from build123d import *

# Parameters (mm, degrees)
SKETCH1_R                  = 5.25
SKETCH1_R_2                = 2.5
BOSS_EXTRUDE1_DEPTH        = 1.6
SKETCH3_W                  = 120
SKETCH3_H                  = 1.6
BOSS_EXTRUDE3_DEPTH        = 60
SKETCH4_R                  = 3
SKETCH4_R_2                = 1.55
SKETCH4_R_3                = 1.75
CUT_EXTRUDE1_DEPTH         = 10
SKETCH6_R                  = 1.7
CUT_EXTRUDE2_DEPTH         = 25
CONVERT_SOLID1_START       = -61
CONVERT_SOLID1_DEPTH       = 122
CONVERT_SOLID1_START_2     = -60
CONVERT_SOLID1_2_DEPTH     = 120
CUT_EXTRUDE3_OUTLINE_W     = 120
CUT_EXTRUDE3_OUTLINE_H     = 60
CUT_EXTRUDE3_OUTLINE_R     = 1.7
CUT_EXTRUDE3_OUTLINE_R_2   = 1.55
CUT_EXTRUDE3_OUTLINE_R_3   = 1.75
CUT_EXTRUDE3_OUTLINE_R_4   = 3
CUT_EXTRUDE3_DEPTH         = 32
CUT_EXTRUDE3_START         = -1.6
CUT_EXTRUDE3_2_OUTLINE_W   = 23.75
CUT_EXTRUDE3_2_OUTLINE_H   = 1.229203673
CUT_EXTRUDE3_2_DEPTH       = 1.6
CUT_EXTRUDE3_3_OUTLINE_W   = 120
CUT_EXTRUDE3_3_OUTLINE_H   = 122.283185308
CUT_EXTRUDE3_3_OUTLINE_W_2 = 23.75
CUT_EXTRUDE3_3_OUTLINE_H_2 = 26.1
CUT_EXTRUDE3_3_OUTLINE_R   = 2.5
CUT_EXTRUDE3_3_OUTLINE_R_2 = 5.25
CUT_EXTRUDE3_3_OUTLINE_R_3 = 1.7
CUT_EXTRUDE3_3_OUTLINE_R_4 = 1.55
CUT_EXTRUDE3_3_OUTLINE_R_5 = 1.75
CUT_EXTRUDE3_3_OUTLINE_R_6 = 3
CUT_EXTRUDE3_3_DEPTH       = 1.6


with BuildPart() as part:
    # Sketch1 → Boss-Extrude1 (new body)
    with BuildSketch(Plane(origin=(0, 0, 0), x_dir=(1, 0, 0), z_dir=(0, 1, 0))):
        Polygon((-60, -12), (-60, 20), (60, 20), (60, -12), (34.5, -12), (11, -12), align=None)
        with Locations(Location((0, 0, 0), (0, 0, 270))):
            Circle(SKETCH1_R, mode=Mode.SUBTRACT)
        with Locations(Location((-43, 0, 0), (0, 0, 270))):
            Circle(SKETCH1_R_2, mode=Mode.SUBTRACT)
        with Locations(Location((43, 0, 0), (0, 0, 90))):
            Circle(SKETCH1_R_2, mode=Mode.SUBTRACT)
    boss_extrude1 = extrude(amount=BOSS_EXTRUDE1_DEPTH)

    # Sketch3 → Boss-Extrude3 (add)
    with BuildSketch(Plane.XZ):
        with Locations((0, 12.8)):
            Rectangle(SKETCH3_W, SKETCH3_H)
    extrude(amount=-BOSS_EXTRUDE3_DEPTH)

    # Mirror1: Boss-Extrude1 across plane
    add(boss_extrude1.mirror(Plane.ZX.offset(30)))

    # Sketch4 → Cut-Extrude1 (cut)
    with BuildSketch(Plane.XY.offset(12)):
        with Locations(Location((22.75, 26.5, 0), (0, 0, 180))):
            Circle(SKETCH4_R)
        with Locations(Location((31.5, 6.5, 0), (0, 0, 180))):
            Circle(SKETCH4_R_2)
        with Locations(Location((14, 6.5, 0), (0, 0, 180))):
            Circle(SKETCH4_R_2)
        with Locations(Location((22.75, 15, 0), (0, 0, 180))):
            Circle(SKETCH4_R_3)
    extrude(amount=CUT_EXTRUDE1_DEPTH, mode=Mode.SUBTRACT)

    # Sketch6 → Cut-Extrude2 (cut)
    with BuildSketch(Plane(origin=(124.244525073, 40.7, 12), x_dir=(1, 0, 0), z_dir=(0, 0, 1))):
        with Locations(Location((-175.244525073, 9.7, 0), (0, 0, 180))):
            Circle(SKETCH6_R)
        with Locations(Location((-146.994525073, 9.7, 0), (0, 0, 180))):
            Circle(SKETCH6_R)
        with Locations(Location((-101.494525073, 9.7, 0), (0, 0, 180))):
            Circle(SKETCH6_R)
        with Locations(Location((-73.244525073, 9.7, 0), (0, 0, 180))):
            Circle(SKETCH6_R)
        with Locations((-175.244525073, -34.5)):
            Circle(SKETCH6_R)
        with Locations((-146.994525073, -34.5)):
            Circle(SKETCH6_R)
        with Locations(Location((-101.494525073, -34.5, 0), (0, 0, 180))):
            Circle(SKETCH6_R)
        with Locations(Location((-73.244525073, -34.5, 0), (0, 0, 180))):
            Circle(SKETCH6_R)
    extrude(amount=CUT_EXTRUDE2_DEPTH, mode=Mode.SUBTRACT)

    # Convert-Solid1: read off the stored shape, not the designer's step
    # Convert-Solid1 outline → Convert-Solid1 (cut)
    with BuildSketch(Plane.YZ.offset(CONVERT_SOLID1_START)):
        with BuildLine():
            Line((60, 13.6), (57.2, 13.6))
            ThreePointArc((57.2, 13.6), (59.179898987, 12.779898987), (60, 10.8))
            Line((60, 10.8), (60, 13.6))
        make_face()
        with BuildLine():
            ThreePointArc((0, 10.8), (0.820101013, 12.779898987), (2.8, 13.6))
            Line((2.8, 13.6), (0, 13.6))
            Line((0, 13.6), (0, 10.8))
        make_face()
    extrude(amount=CONVERT_SOLID1_DEPTH, mode=Mode.SUBTRACT)

    # Convert-Solid1 2 outline → Convert-Solid1 2 (add)
    with BuildSketch(Plane.YZ.offset(CONVERT_SOLID1_START_2)):
        with BuildLine():
            Line((58.4, 12), (57.2, 12))
            ThreePointArc((57.2, 12), (58.048528137, 11.648528137), (58.4, 10.8))
            Line((58.4, 10.8), (58.4, 12))
        make_face()
        with BuildLine():
            ThreePointArc((1.6, 10.8), (1.951471863, 11.648528137), (2.8, 12))
            Line((2.8, 12), (1.6, 12))
            Line((1.6, 12), (1.6, 10.8))
        make_face()
    extrude(amount=CONVERT_SOLID1_2_DEPTH)

    # Cut-Extrude3: read off the stored shape, not the designer's step
    # Cut-Extrude3 outline → Cut-Extrude3 (cut)
    with BuildSketch(Plane(origin=(0, 0, 12), x_dir=(-1, 0, 0), z_dir=(0, 0, -1))):
        with Locations((0, 30)):
            Rectangle(CUT_EXTRUDE3_OUTLINE_W, CUT_EXTRUDE3_OUTLINE_H)
        with Locations((51, 50.4)):
            Circle(CUT_EXTRUDE3_OUTLINE_R, mode=Mode.SUBTRACT)
        with Locations((-51, 6.2)):
            Circle(CUT_EXTRUDE3_OUTLINE_R, mode=Mode.SUBTRACT)
        with Locations((-31.5, 6.5)):
            Circle(CUT_EXTRUDE3_OUTLINE_R_2, mode=Mode.SUBTRACT)
        with Locations((-22.75, 6.2)):
            Circle(CUT_EXTRUDE3_OUTLINE_R, mode=Mode.SUBTRACT)
        with Locations((-14, 6.5)):
            Circle(CUT_EXTRUDE3_OUTLINE_R_2, mode=Mode.SUBTRACT)
        with Locations((-22.75, 15)):
            Circle(CUT_EXTRUDE3_OUTLINE_R_3, mode=Mode.SUBTRACT)
        with Locations((-22.75, 26.5)):
            Circle(CUT_EXTRUDE3_OUTLINE_R_4, mode=Mode.SUBTRACT)
        with Locations((22.75, 6.2)):
            Circle(CUT_EXTRUDE3_OUTLINE_R, mode=Mode.SUBTRACT)
        with Locations((51, 6.2)):
            Circle(CUT_EXTRUDE3_OUTLINE_R, mode=Mode.SUBTRACT)
        with Locations((-51, 50.4)):
            Circle(CUT_EXTRUDE3_OUTLINE_R, mode=Mode.SUBTRACT)
        with Locations((-22.75, 50.4)):
            Circle(CUT_EXTRUDE3_OUTLINE_R, mode=Mode.SUBTRACT)
        with Locations((22.75, 50.4)):
            Circle(CUT_EXTRUDE3_OUTLINE_R, mode=Mode.SUBTRACT)
    extrude(amount=CUT_EXTRUDE3_DEPTH, mode=Mode.SUBTRACT)

    # Cut-Extrude3 2 outline → Cut-Extrude3 2 (cut)
    with BuildSketch(Plane(origin=(0, 0, 12), x_dir=(-1, 0, 0), z_dir=(0, 0, -1)).offset(CUT_EXTRUDE3_START)):
        with Locations((-22.625, 0.614601836)):
            Rectangle(CUT_EXTRUDE3_2_OUTLINE_W, CUT_EXTRUDE3_2_OUTLINE_H)
    extrude(amount=CUT_EXTRUDE3_2_DEPTH, mode=Mode.SUBTRACT)

    # Cut-Extrude3 3 outline → Cut-Extrude3 3 (add)
    with BuildSketch(Plane(origin=(0, 0, 12), x_dir=(-1, 0, 0), z_dir=(0, 0, -1)).offset(CUT_EXTRUDE3_START)):
        with Locations((0, 30)):
            Rectangle(CUT_EXTRUDE3_3_OUTLINE_W, CUT_EXTRUDE3_3_OUTLINE_H)
        with Locations((-22.625, -11.820796327)):
            Rectangle(CUT_EXTRUDE3_3_OUTLINE_W_2, CUT_EXTRUDE3_3_OUTLINE_H_2, mode=Mode.SUBTRACT)
        with Locations((-43, -11.141592654)):
            Circle(CUT_EXTRUDE3_3_OUTLINE_R, mode=Mode.SUBTRACT)
        with Locations((0, -11.141592654)):
            Circle(CUT_EXTRUDE3_3_OUTLINE_R_2, mode=Mode.SUBTRACT)
        with Locations((43, -11.141592654)):
            Circle(CUT_EXTRUDE3_3_OUTLINE_R, mode=Mode.SUBTRACT)
        with Locations((51, 50.4)):
            Circle(CUT_EXTRUDE3_3_OUTLINE_R_3, mode=Mode.SUBTRACT)
        with Locations((-51, 6.2)):
            Circle(CUT_EXTRUDE3_3_OUTLINE_R_3, mode=Mode.SUBTRACT)
        with Locations((-31.5, 6.5)):
            Circle(CUT_EXTRUDE3_3_OUTLINE_R_4, mode=Mode.SUBTRACT)
        with Locations((-22.75, 6.2)):
            Circle(CUT_EXTRUDE3_3_OUTLINE_R_3, mode=Mode.SUBTRACT)
        with Locations((-14, 6.5)):
            Circle(CUT_EXTRUDE3_3_OUTLINE_R_4, mode=Mode.SUBTRACT)
        with Locations((-22.75, 15)):
            Circle(CUT_EXTRUDE3_3_OUTLINE_R_5, mode=Mode.SUBTRACT)
        with Locations((-22.75, 26.5)):
            Circle(CUT_EXTRUDE3_3_OUTLINE_R_6, mode=Mode.SUBTRACT)
        with Locations((22.75, 6.2)):
            Circle(CUT_EXTRUDE3_3_OUTLINE_R_3, mode=Mode.SUBTRACT)
        with Locations((51, 6.2)):
            Circle(CUT_EXTRUDE3_3_OUTLINE_R_3, mode=Mode.SUBTRACT)
        with Locations((-51, 50.4)):
            Circle(CUT_EXTRUDE3_3_OUTLINE_R_3, mode=Mode.SUBTRACT)
        with Locations((-22.75, 50.4)):
            Circle(CUT_EXTRUDE3_3_OUTLINE_R_3, mode=Mode.SUBTRACT)
        with Locations((22.75, 50.4)):
            Circle(CUT_EXTRUDE3_3_OUTLINE_R_3, mode=Mode.SUBTRACT)
        with Locations((43, 71.141592654)):
            Circle(CUT_EXTRUDE3_3_OUTLINE_R, mode=Mode.SUBTRACT)
        with Locations((-43, 71.141592654)):
            Circle(CUT_EXTRUDE3_3_OUTLINE_R, mode=Mode.SUBTRACT)
        with Locations((0, 71.141592654)):
            Circle(CUT_EXTRUDE3_3_OUTLINE_R_2, mode=Mode.SUBTRACT)
    extrude(amount=CUT_EXTRUDE3_3_DEPTH)


solid = part.part
CAD build for the part. Positions are in the model's coordinates, mm. Give positions to 0.01 mm unless a question says otherwise; leave off trailing zeros. Write each loop counter-clockwise with the first axis right and the second up, starting at its lowest first coordinate (ties: lowest second). Pieces come first, ordered by that corner, then holes. Notation, with made-up numbers: (-8.75, 46.5) - (-1.75, 46.5) arc R23 cw to (-1.75, 80.5) - close; hole circle Ø11 at (51.5, 2). An arc over 180 degrees is marked (long way). Answer as CSV lines item,"result".
Q1. Flat gauge pin, fed straight in: pin 1 Ø5 at (x, y) = (14, 6.5) entering from +Z. Where does the tip first touch, or does it go through?
Result set:
pin 1,"z = 13.6"
Q2. Pull direction X, two halves, no side cores. Call faces 1 (the face through (-23.53, 51.91, 12.79)), 2 (the face through (1, 31, 12)): released by +X, released by -X, zero draft, split by the parting line, or undercut.
Result set:
face 1,"undercut"
face 2,"zero draft"
Q3. Drill centre lines: line 1 (Y direction, x = 22.75, z = 13.2); line 2 (Y direction, x = 31.5, z = 13.1); line 3 (Y direction, x = 51, z = 13.15). Where is each one in solid material? Low to high. Write a range as from..to.
Result set:
line 1,"-31.14..-24.87, 1.23..4.5, 7.9..13.25, 16.75..23.5, 29.5..48.7, 52.1..91.14"
line 2,"-31.14..-24.87, 1.23..4.95, 8.05..91.14"
line 3,"-31.14..4.5, 7.9..48.7, 52.1..91.14"
Q4. Band-saw the part on C-C (z = 12.4). State how many separate pieces and enclosed holes the cut face has, and give its area (3 significant figures).
Result set:
separate pieces,"1"
enclosed holes,"19"
area,"13,700 mm²"
Q5. Band-saw the part on B-B (y = 50.4). Give the cut face in (x, z), and give its area (3 significant figures).
Result set:
outline,"(-60, 12) - (-52.7, 12) - (-52.7, 13.6) - (-60, 13.6) - close; (-49.3, 12) - (-24.45, 12) - (-24.45, 13.6) - (-49.3, 13.6) - close; (-21.05, 12) - (21.05, 12) - (21.05, 13.6) - (-21.05, 13.6) - close; (24.45, 12) - (49.3, 12) - (49.3, 13.6) - (24.45, 13.6) - close; (52.7, 12) - (60, 12) - (60, 13.6) - (52.7, 13.6) - close"
area,"170 mm²"
Q6. Band-saw the part on A-A (x = 43). Give the cut face in (y, z).
Result set:
outline,"(-31.14, 12) - (-13.64, 12) - (-13.64, 13.6) - (-31.14, 13.6) - close; (-8.64, 12) - (68.64, 12) - (68.64, 13.6) - (-8.64, 13.6) - close; (73.64, 12) - (91.14, 12) - (91.14, 13.6) - (73.64, 13.6) - close"
Q7. Band-saw the part on D-D (x = 0). Give the cut face in (y, z).
Result set:
outline,"(-31.14, 12) - (-16.39, 12) - (-16.39, 13.6) - (-31.14, 13.6) - close; (-5.89, 12) - (65.89, 12) - (65.89, 13.6) - (-5.89, 13.6) - close; (76.39, 12) - (91.14, 12) - (91.14, 13.6) - (76.39, 13.6) - close"
